Build history of the part. All positions in model axes, mm. A direction names the side the tool comes from. Round coordinates to 2 decimals unless told otherwise and drop trailing zeros. Write each loop counter-clockwise with the first axis right and the second up, starting at its lowest first coordinate (ties: lowest second). Pieces come first, ordered by that corner, then holes.
from build123d import *

# Parameters (mm, degrees)
SKETCH2_W           = 25.5
SKETCH2_H           = 10
BOSS_EXTRUDE1_DEPTH = 1.2
SKETCH4_W           = 6.75
SKETCH4_H           = 7.05
SKETCH4_W_2         = 7.3
SKETCH4_H_2         = 7.4
BOSS_EXTRUDE2_DEPTH = 4.65
SKETCH5_R           = 1.7
BOSS_EXTRUDE3_DEPTH = 4
SKETCH6_W           = 20
SKETCH6_H           = 7.8
BOSS_EXTRUDE4_DEPTH = 1.4


with BuildPart() as part:
    # Sketch2 → Boss-Extrude1 (new body)
    with BuildSketch(Plane(origin=(0, 0, 0), x_dir=(1, 0, 0), z_dir=(0, 1, 0))):
        Rectangle(SKETCH2_W, SKETCH2_H)
    extrude(amount=BOSS_EXTRUDE1_DEPTH)

    # Sketch4 → Boss-Extrude2 (add)
    with BuildSketch(Plane(origin=(0, 1.2, 0), x_dir=(1, 0, 0), z_dir=(0, 1, 0))):
        with Locations((-5.375, 0)):
            Rectangle(SKETCH4_W, SKETCH4_H)
        with Locations((5.65, 0)):
            Rectangle(SKETCH4_W_2, SKETCH4_H_2)
    extrude(amount=BOSS_EXTRUDE2_DEPTH)

    # Sketch5 → Boss-Extrude3 (add)
    with BuildSketch(Plane(origin=(0, 5.85, 0), x_dir=(1, 0, 0), z_dir=(0, 1, 0))):
        with Locations(Location((5.65, 0, 0), (0, 0, 270))):
            Circle(SKETCH5_R)
    extrude(amount=BOSS_EXTRUDE3_DEPTH)

    # Sketch6 → Boss-Extrude4 (add)
    with BuildSketch(Plane.XZ):
        Rectangle(SKETCH6_W, SKETCH6_H)
    extrude(amount=BOSS_EXTRUDE4_DEPTH)


solid = part.part
1) Wall check: L1, parallel to X at y = 4.25, z = -0.25; L2, parallel to Z at x = -6.75, y = -0.25; L3, parallel to Y at x = -5.5, z = 4. Give the ranges that are in metal, low to high.
Results:
L1: x = -8.75 to -2, 2 to 9.3
L2: z = -3.9 to 3.9
L3: y = 0 to 1.2
2) Slice it at B-B (z = 0). Write the cut outline in (x, y).
Results:
outline: (-12.75, 0) - (-10, 0) - (-10, -1.4) - (10, -1.4) - (10, 0) - (12.75, 0) - (12.75, 1.2) - (9.3, 1.2) - (9.3, 5.85) - (7.35, 5.85) - (7.35, 9.85) - (3.95, 9.85) - (3.95, 5.85) - (2, 5.85) - (2, 1.2) - (-2, 1.2) - (-2, 5.85) - (-8.75, 5.85) - (-8.75, 1.2) - (-12.75, 1.2) - close
3) Slice it at A-A (y = 3). Write the cut outline in (x, z) (3 decimals).
Results:
outline: (-8.75, -3.525) - (-2, -3.525) - (-2, 3.525) - (-8.75, 3.525) - close; (2, -3.7) - (9.3, -3.7) - (9.3, 3.7) - (2, 3.7) - close
4) Which spindle directions (+Z, -Z, +X, -X, +Y, -Y) get a long thin tool onto all of the face, cutting with end or side? Do faces 5 (the flat face through (-8.75, 3, 0)), 6 (the flat face through (6, 3, 3.7)), 7 (the flat face through (-5, 3, -3.525)), 8 (the flat face through (10, -1, 0)). Say none if no direction does.
Results:
face 5: +Z, -Z, -X, +Y
face 6: +Z, +X, -X, +Y
face 7: -Z, -X, +Y
face 8: +Z, -Z, +X, -Y
5) Pin check, flat tips, straight feed: pin 1 Ø3.5 at (y, z) = (4.5, -0.5) entering from +X; pin 2 Ø0.7 at (x, y) = (-2, -1) entering from -Z; pin 3 Ø2 at (x, z) = (9, -3.5) entering from +Y. Stop position of each tip, or through.
Results:
pin 1: stops at x = 9.3
pin 2: stops at z = -3.9
pin 3: stops at y = 5.85
6) Mould opens along X. For faces 1 (the flat face through (12.75, 1, 0)), 2 (the cylindrical face through (7.336, 7.822, -0.221)), 3 (the flat face through (-2, 3, 0)), 4 (the flat face through (6, 3, -3.7)) say: released by +X, released by -X, zero draft, split by the parting line, or undercut.
Results:
face 1: released by +X
face 2: split by the parting line
face 3: undercut
face 4: zero draft
7) Slice it at D-D (x = 1.5). Write the cut outline in (y, z), plus the area to 3 significant figures.
Results:
outline: (-1.4, -3.9) - (0, -3.9) - (0, -5) - (1.2, -5) - (1.2, 5) - (0, 5) - (0, 3.9) - (-1.4, 3.9) - close
area: 22.9 mm2
8) Slice it at C-C (x = 5.65). Write the cut outline in (y, z), plus the area to 3 significant figures.
Results:
outline: (-1.4, -3.9) - (0, -3.9) - (0, -5) - (1.2, -5) - (1.2, -3.7) - (5.85, -3.7) - (5.85, -1.7) - (9.85, -1.7) - (9.85, 1.7) - (5.85, 1.7) - (5.85, 3.7) - (1.2, 3.7) - (1.2, 5) - (0, 5) - (0, 3.9) - (-1.4, 3.9) - close
area: 70.9 mm2
